from build123d import *

# Parameters (mm, degrees)
F1_DEPTH = 6.5
F2_DEPTH = 5
F3_R     = 5
F4_W     = 7.6346651632
F4_H     = 12.0459031314
F5_DEPTH = 1


with BuildPart() as f1:
    # F0 (on Front) → F1 (new body)
    with BuildSketch(Plane.XZ):
        Polygon((42.5548888743, 28.6260936409), (31.0699325055, 28.6260936409), (0, 28.6260936409), (-47.5578345358, 17.6459699869), (-47.5578345358, -24.210675411), (-23.4520491213, -32.7111370862), (42.5548888743, -32.7111370862), align=None)
        with BuildLine():
            Line((-19, 12.625), (0, 16.5))
            Line((0, 16.5), (17.5, 16.5))
            ThreePointArc((17.5, 16.5), (34, 0), (17.5, -16.5))
            Line((17.5, -16.5), (0, -16.5))
            Line((0, -16.5), (-19, -12.625))
            Line((-19, -12.625), (-34, -9.65))
            Line((-34, -9.65), (-34, 9.65))
            Line((-34, 9.65), (-19, 12.625))
        make_face(mode=Mode.SUBTRACT)
    extrude(amount=F1_DEPTH)

    # F0 (on Front) → F2 (join)
    with BuildSketch(Plane.XZ):
        Polygon((42.5548888743, 28.6260936409), (31.0699325055, 28.6260936409), (0, 28.6260936409), (-47.5578345358, 17.6459699869), (-47.5578345358, -24.210675411), (-23.4520491213, -32.7111370862), (42.5548888743, -32.7111370862), align=None)
        with BuildLine():
            Line((-19, 12.625), (0, 16.5))
            Line((0, 16.5), (17.5, 16.5))
            ThreePointArc((17.5, 16.5), (34, 0), (17.5, -16.5))
            Line((17.5, -16.5), (0, -16.5))
            Line((0, -16.5), (-19, -12.625))
            Line((-19, -12.625), (-34, -9.65))
            Line((-34, -9.65), (-34, 9.65))
            Line((-34, 9.65), (-19, 12.625))
        make_face(mode=Mode.SUBTRACT)
        with BuildLine():
            Line((17.5, 16.5), (0, 16.5))
            Line((0, 16.5), (-19, 12.625))
            Line((-19, 12.625), (-34, 9.65))
            Line((-34, 9.65), (-34, -9.65))
            Line((-34, -9.65), (-19, -12.625))
            Line((-19, -12.625), (0, -16.5))
            Line((0, -16.5), (17.5, -16.5))
            ThreePointArc((17.5, -16.5), (34, 0), (17.5, 16.5))
        make_face()
    extrude(amount=-F2_DEPTH)

    # F3
    f3_edges = [f1.edges().sort_by_distance(p)[0] for p in [
        (42.554889, -0.75, 28.626094),
        (42.554889, -0.75, -32.711137),
        (-47.557835, -0.75, -24.210675),
        (-47.557835, -0.75, 17.64597),
        (0, -0.75, 28.626094),
        (-23.452049, -0.75, -32.711137),
    ]]
    fillet(f3_edges, radius=F3_R)

    # F4 (on face) → F5 (join)
    with BuildSketch(Plane.XZ.offset(6.5)):
        with Locations((1.6826674184, -23.3507947996)):
            Rectangle(F4_W, F4_H)
    extrude(amount=F5_DEPTH)


solid = f1.part
Geometry check sheet. Reference: the model listing, model coordinates, mm. A direction names the side the tool comes from. Round coordinates to 2 decimals unless told otherwise and drop trailing zeros. Write each loop counter-clockwise with the first axis right and the second up, starting at its lowest first coordinate (ties: lowest second). Pieces come first, ordered by that corner, then holes. Notation, with made-up numbers: (35, 67.5) -> (79, 67.5) arc R28 ccw to (79, 101.5) -> close; hole circle Ø2 at (65, 53.25). An arc over 180 degrees is marked (long way). One line per item, written item: value. Start each with the question number.
(1) Scan lines: line 1 (Y direction, x = -35, z = 18.5); line 2 (Y direction, x = -15.5, z = -4); line 3 (Z direction, x = -31, y = -1.5) (1 decimal). Record each from-to range of solid material in increasing order. Write a range as [from, to].
(2) Access from +Z, -Z, +X, -X, +Y, -Y to the whole of each face (thin tool, end or side, straight path). Record for faces 5 (the cylindrical face through (-46.5, -0.83, 16.744)), 6 (the flat face through (0, 0, 0)).
(3) Cross-section at C-C, the plane y = 1. Record the cut outline in (x, z), and give its area (3 significant figures).
(4) Cross-section at D-D, the plane x = -26.5. Record the cut outline in (y, z).
(5) Cross-section at B-B, the plane z = 0. Record the cut outline in (x, y), and give its area (3 significant figures).
(6) Go/stop test with flat-tipped pins: pin 1 Ø2 at (x, z) = (-35, -22) entering from -Y; pin 2 Ø0.5 at (y, z) = (-7, -25) entering from +X; pin 3 Ø0.8 at (x, y) = (0.5, -7) entering from +Z. Record where each tip stops, or that it passes through.
(7) Cross-section at A-A, the plane y = -4.25. Record the cut outline in (x, z) (3 decimals), and give its area (3 significant figures).
(8) Draft check along Z on faces 1 (the cylindrical face through (41.129, -0.67, -31.208)), 2 (the flat face through (-3, 5, -2)), 3 (the flat face through (9, -3, 16.5)), 4 (the flat face through (9, -3, -16.5)). Enter one of: +Z half, -Z half, draft (parallel to the pull), parting line (faces both ways), or undercut.
Answer:
1. line 1: [-6.5, 5]
1. line 2: [0, 5]
1. line 3: [-30, -10.2], [10.2, 21.5]
2. face 5: +Z, -X, +Y, -Y
2. face 6: -Y
3. outline: (-47.56, -20.67) arc R5 ccw to (-44.22, -25.39) -> (-24.26, -32.43) arc R5 ccw to (-22.6, -32.71) -> (37.55, -32.71) arc R5 ccw to (42.55, -27.71) -> (42.55, 23.63) arc R5 ccw to (37.55, 28.63) -> (0.57, 28.63) arc R5 ccw to (-0.56, 28.5) -> (-43.68, 18.54) arc R5 ccw to (-47.56, 13.67) -> close
3. area: 5,150 mm²
4. outline: (-6.5, -31.64) -> (5, -31.64) -> (5, 22.51) -> (-6.5, 22.51) -> (-6.5, 11.14) -> (0, 11.14) -> (0, -11.14) -> (-6.5, -11.14) -> close
5. outline: (-47.56, -6.5) -> (-34, -6.5) -> (-34, 0) -> (34, 0) -> (34, -6.5) -> (42.55, -6.5) -> (42.55, 5) -> (-47.56, 5) -> close
5. area: 594 mm²
6. pin 1: y = -6.5
6. pin 2: x = 5.5
6. pin 3: z = -17.33
7. outline: (-47.558, -20.672) arc R5 ccw to (-44.221, -25.387) -> (-24.259, -32.427) arc R5 ccw to (-22.596, -32.711) -> (37.555, -32.711) arc R5 ccw to (42.555, -27.711) -> (42.555, 23.626) arc R5 ccw to (37.555, 28.626) -> (0.57, 28.626) arc R5 ccw to (-0.555, 28.498) -> (-43.683, 18.541) arc R5 ccw to (-47.558, 13.669) -> close; hole (-34, -9.65) -> (-19, -12.625) -> (0, -16.5) -> (17.5, -16.5) arc R16.5 ccw to (17.5, 16.5) -> (0, 16.5) -> (-19, 12.625) -> (-34, 9.65) -> close
7. area: 3,250 mm²
8. face 1: -Z half
8. face 2: draft
8. face 3: undercut
8. face 4: undercut
